```python
from build123d import *

# Parameters (mm, degrees)
F0_W     = 104
F0_H     = 24.762767
F0_R     = 2
F1_DEPTH = 2
F2_R     = 1.6
F3_DEPTH = 4


with BuildPart() as f1:
    # F0 (on Top) → F1 (new body)
    with BuildSketch(Plane.XY):
        with Locations((0, -0.776007)):
            Rectangle(F0_W, F0_H)
        with Locations((-48, -9.15739)):
            Circle(F0_R, mode=Mode.SUBTRACT)
        with Locations((48, -9.15739)):
            Circle(F0_R, mode=Mode.SUBTRACT)
        with Locations((-48, 7.605377)):
            Circle(F0_R, mode=Mode.SUBTRACT)
        with Locations((48, 7.605377)):
            Circle(F0_R, mode=Mode.SUBTRACT)
    extrude(amount=F1_DEPTH)

    # F2 (on Front) → F3 (join, symmetric)
    with BuildSketch(Plane.XZ):
        with BuildLine():
            Line((-28, 20), (-28, 0))
            Line((-28, 0), (-20, 0))
            Line((-20, 0), (-20, 20))
            ThreePointArc((-20, 20), (-24, 16), (-28, 20))
        make_face()
        with BuildLine():
            ThreePointArc((-20, 20), (-24, 24), (-28, 20))
            ThreePointArc((-28, 20), (-24, 16), (-20, 20))
        make_face()
        with Locations((-24, 20)):
            Circle(F2_R, mode=Mode.SUBTRACT)
        with BuildLine():
            Line((20, 20), (20, 0))
            Line((20, 0), (28, 0))
            Line((28, 0), (28, 20))
            ThreePointArc((28, 20), (24, 16), (20, 20))
        make_face()
        with BuildLine():
            ThreePointArc((28, 20), (24, 24), (20, 20))
            ThreePointArc((20, 20), (24, 16), (28, 20))
        make_face()
        with Locations((24, 20)):
            Circle(F2_R, mode=Mode.SUBTRACT)
        with BuildLine():
            Line((-44, 20), (-44, 0))
            Line((-44, 0), (-36, 0))
            Line((-36, 0), (-36, 20))
            ThreePointArc((-36, 20), (-40, 16), (-44, 20))
        make_face()
        with BuildLine():
            ThreePointArc((-36, 20), (-40, 24), (-44, 20))
            ThreePointArc((-44, 20), (-40, 16), (-36, 20))
        make_face()
        with Locations((-40, 20)):
            Circle(F2_R, mode=Mode.SUBTRACT)
        with BuildLine():
            Line((-12, 20), (-12, 0))
            Line((-12, 0), (-4, 0))
            Line((-4, 0), (-4, 20))
            ThreePointArc((-4, 20), (-8, 16), (-12, 20))
        make_face()
        with BuildLine():
            ThreePointArc((-4, 20), (-8, 24), (-12, 20))
            ThreePointArc((-12, 20), (-8, 16), (-4, 20))
        make_face()
        with Locations((-8, 20)):
            Circle(F2_R, mode=Mode.SUBTRACT)
        with BuildLine():
            Line((4, 20), (4, 0))
            Line((4, 0), (12, 0))
            Line((12, 0), (12, 20))
            ThreePointArc((12, 20), (8, 16), (4, 20))
        make_face()
        with BuildLine():
            ThreePointArc((12, 20), (8, 24), (4, 20))
            ThreePointArc((4, 20), (8, 16), (12, 20))
        make_face()
        with Locations((8, 20)):
            Circle(F2_R, mode=Mode.SUBTRACT)
        with BuildLine():
            Line((36, 20), (36, 0))
            Line((36, 0), (44, 0))
            Line((44, 0), (44, 20))
            ThreePointArc((44, 20), (40, 16), (36, 20))
        make_face()
        with BuildLine():
            ThreePointArc((44, 20), (40, 24), (36, 20))
            ThreePointArc((36, 20), (40, 16), (44, 20))
        make_face()
        with Locations((40, 20)):
            Circle(F2_R, mode=Mode.SUBTRACT)
    extrude(amount=F3_DEPTH, both=True)


solid = f1.part
```
Part model, mm, in its own coordinate system. A direction names the side the tool comes from. Coordinates: 2 decimals unless noted, no trailing zeros. Write each loop counter-clockwise with the first axis right and the second up, starting at its lowest first coordinate (ties: lowest second). Pieces come first, ordered by that corner, then holes.
Item 1: Slice it at A-A (x = -8). Write the cut outline in (y, z), and give its area (3 significant figures).
Item 2: Mould opens along Z. For faces 5 (the face through (7.792, 0.056, 21.586)), 6 (the face through (-24, 4, 13)), 7 (the face through (40, 0, 24)), 8 (the face through (-40.208, 0.056, 21.586)) say: released by +Z, released by -Z, zero draft, split by the parting line, or undercut.
Item 3: Slice it at C-C (y = 1.5). Count the separate pieces of the cut face and the enclosed holes in it, and give its area (3 significant figures).
Item 4: Probe line 1 (X direction, y = -1.5, z = 7.75); line 2 (Y direction, x = -48, z = 1.05); line 3 (Z direction, x = 24, y = 0.25). List the from-to ranges inside material, lowest first.
Item 5: Slice it at B-B (z = 7.5). Write the cut outline in (x, y).
Item 6: Slice it at D-D (x = 48). Write the cut outline in (y, z), and give its area (3 significant figures).
Item 7: Which spindle directions (+Z, -Z, +X, -X, +Y, -Y) get a long thin tool onto all of the face, cutting with end or side? Do faces 1 (the face through (-40, -4, 13)), 2 (the face through (4, 0, 11)), 3 (the face through (40, 4, 13)), 4 (the face through (-44, 0, 11)). Say none if no direction does.
Item 8: Pin check, flat tips, straight feed: pin 1 (6 mm diameter, centred on y = -6, z = 17.5, fed in from -X); pin 2 (4 mm diameter, centred on x = -42, z = 8, fed in from -Y); pin 3 (1.5 mm diameter, centred on y = 2, z = 11, fed in from +X). Stop position of each tip, or through.
Results found:
1. outline: (-13.16, 0) - (11.61, 0) - (11.61, 2) - (4, 2) - (4, 18.4) - (-4, 18.4) - (-4, 2) - (-13.16, 2) - close; (-4, 21.6) - (4, 21.6) - (4, 24) - (-4, 24) - close
1. area: 200 mm2
2. face 5: undercut
2. face 6: zero draft
2. face 7: released by +Z
2. face 8: undercut
3. separate pieces: 1
3. enclosed holes: 6
3. area: 1,170 mm2
4. line 1: x = -44 to -36, -28 to -20, -12 to -4, 4 to 12, 20 to 28, 36 to 44
4. line 2: y = -13.16 to -11.16, -7.16 to 5.61, 9.61 to 11.61
4. line 3: z = 0 to 18.4, 21.6 to 24
5. outline: (-44, -4) - (-36, -4) - (-36, 4) - (-44, 4) - close; (-28, -4) - (-20, -4) - (-20, 4) - (-28, 4) - close; (-12, -4) - (-4, -4) - (-4, 4) - (-12, 4) - close; (4, -4) - (12, -4) - (12, 4) - (4, 4) - close; (20, -4) - (28, -4) - (28, 4) - (20, 4) - close; (36, -4) - (44, -4) - (44, 4) - (36, 4) - close
6. outline: (-13.16, 0) - (-11.16, 0) - (-11.16, 2) - (-13.16, 2) - close; (-7.16, 0) - (5.61, 0) - (5.61, 2) - (-7.16, 2) - close; (9.61, 0) - (11.61, 0) - (11.61, 2) - (9.61, 2) - close
6. area: 33.5 mm2
7. face 1: +Z, +X, -X, -Y
7. face 2: +Z, +Y, -Y
7. face 3: +Z, +X, -X, +Y
7. face 4: +Z, -X, +Y, -Y
8. pin 1: stops at x = -44
8. pin 2: stops at y = -4
8. pin 3: stops at x = 44
